from build123d import *

# Parameters (mm, degrees)
F1_DEPTH = 12
F2_R     = 3
F3_DEPTH = 37.501
F4_R     = 3
F5_DEPTH = 37.501
F6_R     = 5


with BuildPart() as f1:
    # F0 (on Top) → F1 (new body)
    with BuildSketch(Plane.XY):
        Polygon((-16.078127, 165.7075), (-41.078127, 165.7075), (-41.078127, 152.7075), (-53.578127, 152.7075), (-53.578127, -41.2925), (-41.078127, -41.2925), (-41.078127, -54.2925), (-16.078127, -54.2925), (-16.078127, -41.2925), (-3.578127, -41.2925), (-3.578127, 152.7075), (-16.078127, 152.7075), align=None)
    extrude(amount=F1_DEPTH)

    # F2 (on face) → F3 (cut, through all)
    with BuildSketch(Plane(origin=(-41.078127, 0, 0), x_dir=(0, -1, 0), z_dir=(-1, 0, 0))):
        with Locations((-159.2075, 6)):
            Circle(F2_R)
    extrude(amount=-F3_DEPTH, mode=Mode.SUBTRACT)

    # F4 (on face) → F5 (cut, through all)
    with BuildSketch(Plane(origin=(-41.078127, 0, 0), x_dir=(0, -1, 0), z_dir=(-1, 0, 0))):
        with Locations((47.7925, 6)):
            Circle(F4_R)
    extrude(amount=-F5_DEPTH, mode=Mode.SUBTRACT)

    # F6
    f6_edges = [f1.edges().sort_by_distance(p)[0] for p in [
        (-28.578127, -54.2925, 12),
        (-28.578127, -54.2925, 0),
        (-28.578127, 165.7075, 12),
        (-28.578127, 165.7075, 0),
        (-3.578127, 152.7075, 6),
        (-53.578127, 152.7075, 6),
        (-53.578127, -41.2925, 6),
        (-3.578127, -41.2925, 6),
    ]]
    fillet(f6_edges, radius=F6_R)


solid = f1.part
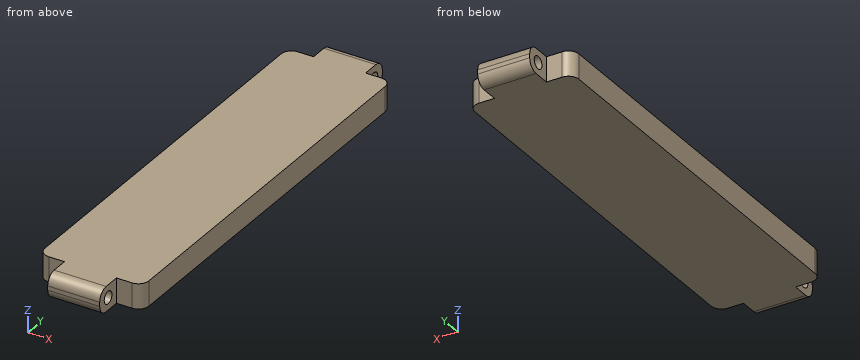
The model under review builds one solid part; all positions refer to its coordinate system, in mm. Give positions to 0.01 mm unless a question says otherwise; leave off trailing zeros. Write each loop counter-clockwise with the first axis right and the second up, starting at its lowest first coordinate (ties: lowest second). Pieces come first, ordered by that corner, then holes.
1. For P1, Ø2, axis at x = -13, z = 5.5, coming from the +Y side; P2, Ø6, axis at x = -46.5, z = 3, coming from the -Y side; P3, Ø6, axis at y = -47, z = 8.5, coming from the -X side, all flat-tipped, find the tip position at first contact; note any pin that passes through.
2. Add section B-B, the plane x = -11. Write out the cut boundary in (y, z).
3. Wall thickness on L1, parallel to Y at x = -24, z = 5.75; L2, parallel to Y at x = -26, z = 7.75; L3, parallel to Y at x = -45.5, z = 5: over which ranges is each line inside the solid? List them lowest first.
4. Add section A-A, the plane x = -30. Write out the cut boundary in (y, z), plus the area to 3 significant figures.
Worked answers:
1. P1: stops at y = 152.71
1. P2: stops at y = -41.29
1. P3: stops at x = -41.08
2. outline: (-41.29, 0) - (152.71, 0) - (152.71, 12) - (-41.29, 12) - close
3. L1: y = -54.29 to -50.78, -44.8 to 156.22, 162.2 to 165.71
3. L2: y = -54.24 to -50.23, -45.36 to 156.77, 161.64 to 165.65
3. L3: y = -41.29 to 152.71
4. outline: (-54.29, 5) arc R5 ccw to (-49.29, 0) - (160.71, 0) arc R5 ccw to (165.71, 5) - (165.71, 7) arc R5 ccw to (160.71, 12) - (-49.29, 12) arc R5 ccw to (-54.29, 7) - close; hole circle Ø6 at (-47.79, 6); hole circle Ø6 at (159.21, 6)
4. area: 2,560 mm2
